Design review of the part built by this model. Coordinates are the model's own, in mm. Coordinates: 2 decimals unless noted, no trailing zeros. Write each loop counter-clockwise with the first axis right and the second up, starting at its lowest first coordinate (ties: lowest second). Pieces come first, ordered by that corner, then holes.
Q1. The part is to be moulded in two halves that separate along X. For faces 1 (the flat face through (-1, 0, 100)), 2 (the cylindrical face through (47.83, 0.11, 40.24)), 3 (the flat face through (-100, 0, -1)), 4 (the cylindrical face through (-52.17, 0.11, 40.24)), say which applies: released by +X, released by -X, zero draft, split by the parting line, or undercut.
Q2. Take a section at B-B, the plane x = -50. Write out the cut boundary in (y, z).
Q3. Take a section at C-C, the plane y = -1.5. Write out the cut boundary in (x, z).
Q4. For L1, parallel to Z at x = -50, y = 4.75; L2, parallel to X at y = 0.5, z = -47.5; L3, parallel to X at y = -1.25, z = -56.5, list the stretches that pass through material, from the lowest coordinate up.
Q5. Take a section at A-A, the plane z = 50. Write out the cut boundary in (x, y), plus the area to 3 significant figures.
from build123d import *

# Parameters (mm, degrees)
F0_W     = 200
F0_H     = 200
F0_R     = 10
F1_DEPTH = 7.5


with BuildPart() as f1:
    # F0 (on Front) → F1 (new body, symmetric)
    with BuildSketch(Plane.XZ):
        Rectangle(F0_W, F0_H)
        with Locations((-50, -50)):
            Circle(F0_R, mode=Mode.SUBTRACT)
        with Locations((50, -50)):
            Circle(F0_R, mode=Mode.SUBTRACT)
        with Locations((-50, 50)):
            Circle(F0_R, mode=Mode.SUBTRACT)
        with Locations((50, 50)):
            Circle(F0_R, mode=Mode.SUBTRACT)
    extrude(amount=F1_DEPTH, both=True)


solid = f1.part
Responses:
1. face 1: zero draft
1. face 2: undercut
1. face 3: released by -X
1. face 4: undercut
2. outline: (-7.5, -100) - (7.5, -100) - (7.5, -60) - (-7.5, -60) - close; (-7.5, -40) - (7.5, -40) - (7.5, 40) - (-7.5, 40) - close; (-7.5, 60) - (7.5, 60) - (7.5, 100) - (-7.5, 100) - close
3. outline: (-100, -100) - (100, -100) - (100, 100) - (-100, 100) - close; hole circle Ø20 at (-50, -50); hole circle Ø20 at (-50, 50); hole circle Ø20 at (50, -50); hole circle Ø20 at (50, 50)
4. L1: z = -100 to -60, -40 to 40, 60 to 100
4. L2: x = -100 to -59.68, -40.32 to 40.32, 59.68 to 100
4. L3: x = -100 to -57.6, -42.4 to 42.4, 57.6 to 100
5. outline: (-100, -7.5) - (-60, -7.5) - (-60, 7.5) - (-100, 7.5) - close; (-40, -7.5) - (40, -7.5) - (40, 7.5) - (-40, 7.5) - close; (60, -7.5) - (100, -7.5) - (100, 7.5) - (60, 7.5) - close
5. area: 2,400 mm2
